from build123d import *

# Parameters (mm, degrees)
BOSS_EXTRUDE1_START = -0.2
SKETCH1_R           = 1.6
BOSS_EXTRUDE1_DEPTH = 7.520002
BOSS_EXTRUDE2_START = -0.2
SKETCH1_7_R         = 1.6
SKETCH1_7_R_2       = 1.995
SKETCH1_7_R_3       = 4.175
SKETCH1_7_R_4       = 1.845
BOSS_EXTRUDE2_DEPTH = 2
BOSS_EXTRUDE3_START = 7.320002
SKETCH1_8_R         = 1.6
BOSS_EXTRUDE3_DEPTH = 11.720001513


with BuildPart() as part:
    # Sketch1 → Boss-Extrude1 (new body)
    with BuildSketch(Plane(origin=(-6551.301651172, 0, 0), x_dir=(0, 0, -1), z_dir=(1, 0, 0)).offset(BOSS_EXTRUDE1_START)):
        with BuildLine():
            Line((783.267150495, -3133.594839225), (763.752150495, -3133.594839225))
            Line((763.752150495, -3133.594839225), (763.752150495, -3135.038892457))
            ThreePointArc((763.752150495, -3135.038892457), (763.664167085, -3135.972751667), (763.403313286, -3136.873745229))
            ThreePointArc((763.403313286, -3136.873745229), (766.079771865, -3141.73149117), (770.352150495, -3138.194839225))
            Line((770.352150495, -3138.194839225), (770.352150495, -3137.594839225))
            ThreePointArc((770.352150495, -3137.594839225), (770.937936933, -3136.180625663), (772.352150495, -3135.594839225))
            Line((772.352150495, -3135.594839225), (783.067150495, -3135.594839225))
            ThreePointArc((783.067150495, -3135.594839225), (790.138218307, -3132.665907037), (793.067150495, -3125.594839225))
            Line((793.067150495, -3125.594839225), (793.067150495, -3121.390787525))
            ThreePointArc((793.067150495, -3121.390787525), (797.458109686, -3116.126374636), (792.467150495, -3111.426918067))
            Line((792.467150495, -3111.426918067), (785.267150495, -3111.426918067))
            ThreePointArc((785.267150495, -3111.426918067), (787.593812026, -3113.342477046), (788.467150495, -3116.226918067))
            Line((788.467150495, -3116.226918067), (788.467150495, -3128.394839225))
            ThreePointArc((788.467150495, -3128.394839225), (786.944105758, -3132.071794487), (783.267150495, -3133.594839225))
        make_face()
        with Locations(Location((766.752150495, -3138.194839225, 0), (0, 0, 180))):
            Circle(SKETCH1_R, mode=Mode.SUBTRACT)
        with Locations(Location((792.467150495, -3116.426918067, 0), (0, 0, 180))):
            Circle(SKETCH1_R, mode=Mode.SUBTRACT)
    extrude(amount=BOSS_EXTRUDE1_DEPTH)

    # Sketch1<7> → Boss-Extrude2 (add)
    with BuildSketch(Plane(origin=(-6551.301651172, 0, 0), x_dir=(0, 0, -1), z_dir=(1, 0, 0)).offset(BOSS_EXTRUDE2_START)):
        with BuildLine():
            Line((792.467150495, -3111.426918067), (785.267150495, -3111.426918067))
            ThreePointArc((785.267150495, -3111.426918067), (786.906779124, -3112.513011303), (788.025771185, -3114.130366343))
            ThreePointArc((788.025771185, -3114.130366343), (789.867415761, -3112.155925289), (792.467150495, -3111.426918067))
        make_face()
        with BuildLine():
            ThreePointArc((797.467150495, -3116.426918067), (796.002684401, -3112.891384161), (792.467150495, -3111.426918067))
            ThreePointArc((792.467150495, -3111.426918067), (789.867415761, -3112.155925289), (788.025771185, -3114.130366343))
            ThreePointArc((788.025771185, -3114.130366343), (788.355609377, -3115.155663565), (788.467150495, -3116.226918067))
            Line((788.467150495, -3116.226918067), (788.467150495, -3118.759075354))
            Line((788.467150495, -3118.759075354), (789.349993208, -3119.641918067))
            Line((789.349993208, -3119.641918067), (793.267150495, -3119.641918067))
            Line((793.267150495, -3119.641918067), (793.267150495, -3121.362503138))
            ThreePointArc((793.267150495, -3121.362503138), (796.275037048, -3119.667288416), (797.467150495, -3116.426918067))
        make_face()
        with Locations(Location((792.467150495, -3116.426918067, 0), (0, 0, 180))):
            Circle(SKETCH1_7_R, mode=Mode.SUBTRACT)
        with BuildLine():
            ThreePointArc((788.025771185, -3114.130366343), (787.802673468, -3114.626180978), (787.634729413, -3115.143287871))
            ThreePointArc((787.634729413, -3115.143287871), (787.733922547, -3115.681072451), (787.767150495, -3116.226918067))
            Line((787.767150495, -3116.226918067), (787.767150495, -3118.132790278))
            ThreePointArc((787.767150495, -3118.132790278), (788.069288323, -3118.805743053), (788.467150495, -3119.426918067))
            Line((788.467150495, -3119.426918067), (788.467150495, -3118.759075354))
            Line((788.467150495, -3118.759075354), (788.467150495, -3116.226918067))
            ThreePointArc((788.467150495, -3116.226918067), (788.355609377, -3115.155663565), (788.025771185, -3114.130366343))
        make_face()
        with BuildLine():
            Line((788.467150495, -3118.759075354), (788.467150495, -3119.426918067))
            ThreePointArc((788.467150495, -3119.426918067), (790.503939908, -3121.025374785), (793.067150495, -3121.390787525))
            ThreePointArc((793.067150495, -3121.390787525), (793.167293339, -3121.377655385), (793.267150495, -3121.362503138))
            Line((793.267150495, -3121.362503138), (793.267150495, -3119.641918067))
            Line((793.267150495, -3119.641918067), (789.349993208, -3119.641918067))
            Line((789.349993208, -3119.641918067), (788.467150495, -3118.759075354))
        make_face()
        with BuildLine():
            Line((788.467150495, -3119.426918067), (788.467150495, -3125.924760779))
            Line((788.467150495, -3125.924760779), (789.349993208, -3125.041918067))
            Line((789.349993208, -3125.041918067), (793.067150495, -3125.041918067))
            Line((793.067150495, -3125.041918067), (793.067150495, -3121.390787525))
            ThreePointArc((793.067150495, -3121.390787525), (790.503939908, -3121.025374785), (788.467150495, -3119.426918067))
        make_face()
        with BuildLine():
            Line((783.267150495, -3133.594839225), (763.752150495, -3133.594839225))
            Line((763.752150495, -3133.594839225), (763.752150495, -3135.038892457))
            ThreePointArc((763.752150495, -3135.038892457), (763.664167085, -3135.972751667), (763.403313286, -3136.873745229))
            ThreePointArc((763.403313286, -3136.873745229), (766.079771865, -3141.73149117), (770.352150495, -3138.194839225))
            Line((770.352150495, -3138.194839225), (770.352150495, -3137.594839225))
            ThreePointArc((770.352150495, -3137.594839225), (770.937936933, -3136.180625663), (772.352150495, -3135.594839225))
            Line((772.352150495, -3135.594839225), (783.067150495, -3135.594839225))
            ThreePointArc((783.067150495, -3135.594839225), (790.138218307, -3132.665907037), (793.067150495, -3125.594839225))
            Line((793.067150495, -3125.594839225), (793.067150495, -3125.041918067))
            Line((793.067150495, -3125.041918067), (789.349993208, -3125.041918067))
            Line((789.349993208, -3125.041918067), (788.467150495, -3125.924760779))
            Line((788.467150495, -3125.924760779), (788.467150495, -3128.394839225))
            ThreePointArc((788.467150495, -3128.394839225), (786.944105758, -3132.071794487), (783.267150495, -3133.594839225))
        make_face()
        with Locations(Location((766.752150495, -3138.194839225, 0), (0, 0, 180))):
            Circle(SKETCH1_7_R, mode=Mode.SUBTRACT)
        with BuildLine():
            Line((763.752150495, -3111.726918067), (763.752150495, -3132.894839225))
            Line((763.752150495, -3132.894839225), (783.267150495, -3132.894839225))
            ThreePointArc((783.267150495, -3132.894839225), (786.449131011, -3131.57681974), (787.767150495, -3128.394839225))
            Line((787.767150495, -3128.394839225), (787.767150495, -3118.132790278))
            ThreePointArc((787.767150495, -3118.132790278), (787.472048486, -3116.648177904), (787.634729413, -3115.143287871))
            ThreePointArc((787.634729413, -3115.143287871), (786.039664167, -3112.682462123), (783.267150495, -3111.726918067))
            Line((783.267150495, -3111.726918067), (763.752150495, -3111.726918067))
        make_face()
        with Locations((766.097150495, -3122.341918067)):
            Circle(SKETCH1_7_R_2, mode=Mode.SUBTRACT)
        with Locations(Location((777.347150495, -3122.341918067, 0), (0, 0, 180))):
            Circle(SKETCH1_7_R_3, mode=Mode.SUBTRACT)
        with BuildLine():
            Line((763.752150495, -3132.894839225), (763.752150495, -3133.594839225))
            Line((763.752150495, -3133.594839225), (783.267150495, -3133.594839225))
            ThreePointArc((783.267150495, -3133.594839225), (786.944105758, -3132.071794487), (788.467150495, -3128.394839225))
            Line((788.467150495, -3128.394839225), (788.467150495, -3125.924760779))
            Line((788.467150495, -3125.924760779), (788.467150495, -3119.426918067))
            ThreePointArc((788.467150495, -3119.426918067), (788.069288323, -3118.805743053), (787.767150495, -3118.132790278))
            Line((787.767150495, -3118.132790278), (787.767150495, -3128.394839225))
            ThreePointArc((787.767150495, -3128.394839225), (786.449131011, -3131.57681974), (783.267150495, -3132.894839225))
            Line((783.267150495, -3132.894839225), (763.752150495, -3132.894839225))
        make_face()
        with BuildLine():
            Line((763.752150495, -3111.426918067), (763.752150495, -3111.726918067))
            Line((763.752150495, -3111.726918067), (783.267150495, -3111.726918067))
            ThreePointArc((783.267150495, -3111.726918067), (786.039664167, -3112.682462123), (787.634729413, -3115.143287871))
            ThreePointArc((787.634729413, -3115.143287871), (787.802673468, -3114.626180978), (788.025771185, -3114.130366343))
            ThreePointArc((788.025771185, -3114.130366343), (786.906779124, -3112.513011303), (785.267150495, -3111.426918067))
            Line((785.267150495, -3111.426918067), (763.752150495, -3111.426918067))
        make_face()
        with BuildLine():
            ThreePointArc((787.767150495, -3116.226918067), (787.733922547, -3115.681072451), (787.634729413, -3115.143287871))
            ThreePointArc((787.634729413, -3115.143287871), (787.472048486, -3116.648177904), (787.767150495, -3118.132790278))
            Line((787.767150495, -3118.132790278), (787.767150495, -3116.226918067))
        make_face()
        with Locations((766.097150495, -3122.341918067)):
            Circle(SKETCH1_7_R_2)
        with Locations((766.097150495, -3122.341918067)):
            Circle(SKETCH1_7_R_4, mode=Mode.SUBTRACT)
        with Locations((766.097150495, -3122.341918067)):
            Circle(SKETCH1_7_R_4)
    extrude(amount=-BOSS_EXTRUDE2_DEPTH)

    # Sketch1<8> → Boss-Extrude3 (add)
    with BuildSketch(Plane(origin=(-6551.301651172, 0, 0), x_dir=(0, 0, -1), z_dir=(1, 0, 0)).offset(BOSS_EXTRUDE3_START)):
        with BuildLine():
            Line((783.267150495, -3133.594839225), (763.752150495, -3133.594839225))
            Line((763.752150495, -3133.594839225), (763.752150495, -3135.038892457))
            ThreePointArc((763.752150495, -3135.038892457), (763.664167085, -3135.972751667), (763.403313286, -3136.873745229))
            ThreePointArc((763.403313286, -3136.873745229), (766.079771865, -3141.73149117), (770.352150495, -3138.194839225))
            Line((770.352150495, -3138.194839225), (770.352150495, -3137.594839225))
            ThreePointArc((770.352150495, -3137.594839225), (770.937936933, -3136.180625663), (772.352150495, -3135.594839225))
            Line((772.352150495, -3135.594839225), (783.067150495, -3135.594839225))
            ThreePointArc((783.067150495, -3135.594839225), (790.138218307, -3132.665907037), (793.067150495, -3125.594839225))
            Line((793.067150495, -3125.594839225), (793.067150495, -3125.041918067))
            Line((793.067150495, -3125.041918067), (789.349993208, -3125.041918067))
            Line((789.349993208, -3125.041918067), (788.467150495, -3125.924760779))
            Line((788.467150495, -3125.924760779), (788.467150495, -3128.394839225))
            ThreePointArc((788.467150495, -3128.394839225), (786.944105758, -3132.071794487), (783.267150495, -3133.594839225))
        make_face()
        with Locations((766.752150495, -3138.194839225)):
            Circle(SKETCH1_8_R, mode=Mode.SUBTRACT)
        with BuildLine():
            Line((792.467150495, -3111.426918067), (785.267150495, -3111.426918067))
            ThreePointArc((785.267150495, -3111.426918067), (787.593812026, -3113.342477046), (788.467150495, -3116.226918067))
            Line((788.467150495, -3116.226918067), (788.467150495, -3118.759075354))
            Line((788.467150495, -3118.759075354), (789.349993208, -3119.641918067))
            Line((789.349993208, -3119.641918067), (793.267150495, -3119.641918067))
            Line((793.267150495, -3119.641918067), (793.267150495, -3121.362503138))
            ThreePointArc((793.267150495, -3121.362503138), (797.451020747, -3116.025623511), (792.467150495, -3111.426918067))
        make_face()
        with Locations((792.467150495, -3116.426918067)):
            Circle(SKETCH1_8_R, mode=Mode.SUBTRACT)
    extrude(amount=BOSS_EXTRUDE3_DEPTH)


solid = part.part
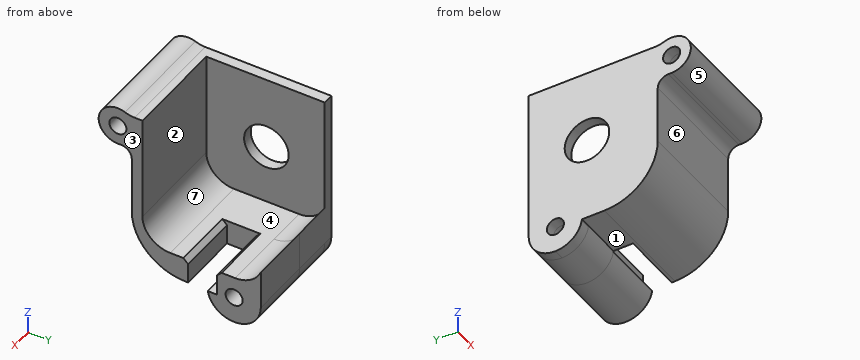
Geometry: final body of the model. Coordinates: model frame, mm. Face numbers are marked on the shaded views. A direction names the side the tool comes from. Give positions to 0.01 mm unless a question says otherwise; leave off trailing zeros. Write each loop counter-clockwise with the first axis right and the second up, starting at its lowest first coordinate (ties: lowest second). Pieces come first, ordered by that corner, then holes. Notation, with made-up numbers: M 89.25,31.25 L 134.25,31.25 A14 cw 134.25,52.25 Z; hole C 56.5,67.5 d4. An arc over 180 degrees is marked long. Answer in a Markdown table with one row per item. Add a question column.
(1) Section B-B on z = -775.5. Return loops of the section in (x, y), and give its area (3 significant figures).
(2) Ray query, line 1 (Y direction, x = -6550, z = -780); line 2 (Y direction, x = -6551.25, z = -787.5); line 3 (X direction, y = -3115, z = -784). Return the intervals inside material, ascending.
(3) Mould query, pull axis Y, two halves, no side actions, for the marked faces 5, 6 and 7. Classes: +Y half, -Y half, draft (parallel to the pull), parting line (faces both ways), or undercut.
(4) Section C-C on x = -6547.25. Return loops of the section in (y, z).
(5) First-contact query: pin 1 (3 mm diameter, centred on x = -6546, z = -777, fed in from -Y); pin 2 (3 mm diameter, centred on y = -3138.19, z = -766.75, fed in from +X); pin 3 (4 mm diameter, centred on x = -6542, z = -778, fed in from +Y); pin 4 (5 mm diameter, centred on x = -6548, y = -3122.5, fed in from +Z). Flat tips, straight axial feed; report the tip coordinate or a pass-through.
(6) Section A-A on x = -6540.5. Return loops of the section in (y, z).
(7) Section D-D on y = -3123. Return loops of the section in (x, z).
(8) Reachability of the marked faces 1, 2, 3 and 4 from +Z, -Z, +X, -X, +Y, -Y: full face, straight path, thin tool, end or side. Return the list, or none.
Result set:
| question | item | result |
|---|---|---|
| 1 | outline | M -6553.5,-3135.59 L -6532.26,-3135.59 L -6532.26,-3133.59 L -6551.5,-3133.59 L -6551.5,-3126.09 L -6553.5,-3126.09 Z; M -6553.5,-3118.6 L -6551.5,-3118.6 L -6551.5,-3111.43 L -6553.5,-3111.43 Z |
| 1 | area | 71.8 mm^2 |
| 2 | line 1 | y = -3135.59 to -3133.59 |
| 2 | line 2 | y = -3134.56 to -3131.42, -3113.21 to -3111.43 |
| 2 | line 3 | x = -6553.5 to -6551.5 |
| 3 | face 5 | parting line |
| 3 | face 6 | -Y half |
| 3 | face 7 | undercut |
| 4 | outline | M -3138.19,-770.35 L -3137.59,-770.35 A2 cw -3135.59,-772.35 L -3135.59,-783.07 A10 ccw -3125.59,-793.07 L -3121.39,-793.07 A5 ccw -3111.43,-792.47 L -3111.43,-785.27 A5.2 cw -3116.23,-788.47 L -3128.39,-788.47 A5.2 cw -3133.59,-783.27 L -3133.59,-763.75 L -3135.04,-763.75 A5 cw -3136.87,-763.4 A3.6 ccw long Z; hole C -3138.19,-766.75 d3.2; hole C -3116.43,-792.47 d3.2 |
| 5 | pin 1 | stops at y = -3135.59 |
| 5 | pin 2 | passes through |
| 5 | pin 3 | stops at y = -3133.59 |
| 5 | pin 4 | stops at z = -788.47 |
| 6 | outline | M -3138.19,-770.35 L -3137.59,-770.35 A2 cw -3135.59,-772.35 L -3135.59,-783.07 A10 ccw -3125.59,-793.07 L -3125.04,-793.07 L -3125.04,-789.35 L -3125.92,-788.47 L -3128.39,-788.47 A5.2 cw -3133.59,-783.27 L -3133.59,-763.75 L -3135.04,-763.75 A5 cw -3136.87,-763.4 A3.6 ccw long Z; M -3121.36,-793.27 A5 ccw -3111.43,-792.47 L -3111.43,-785.27 A5.2 cw -3116.23,-788.47 L -3118.76,-788.47 L -3119.64,-789.35 L -3119.64,-793.27 Z; hole C -3138.19,-766.75 d3.2; hole C -3116.43,-792.47 d3.2 |
| 7 | outline | M -6553.5,-793.07 L -6543.98,-793.07 L -6543.98,-788.47 L -6551.5,-788.47 L -6551.5,-781.47 L -6553.5,-781.47 Z; M -6553.5,-773.22 L -6551.5,-773.22 L -6551.5,-763.75 L -6553.5,-763.75 Z |
| 8 | face 1 | -Z, +X, -X, -Y |
| 8 | face 2 | +Z, +X, +Y |
| 8 | face 3 | +Z, -Z, +X, +Y, -Y |
| 8 | face 4 | +Z, +X |
